```python
from build123d import *

# Parameters (mm, degrees)
ESQUISSE1_R        = 15
ESQUISSE1_R_2      = 3
BOSS_EXTRU_1_DEPTH = 12
CHANFREIN1_SIZE    = 6
CONG_1_R           = 2


with BuildPart() as part:
    # Esquisse1 → Boss.-Extru.1 (new body)
    with BuildSketch(Plane.XY):
        Circle(ESQUISSE1_R)
        Circle(ESQUISSE1_R_2, mode=Mode.SUBTRACT)
    extrude(amount=BOSS_EXTRU_1_DEPTH)

    # Chanfrein1
    chanfrein1_edges = [part.edges().sort_by_distance(p)[0] for p in [
        (-3, 0, 12),
    ]]
    chamfer(chanfrein1_edges, length=CHANFREIN1_SIZE)

    # Congé1
    cong_1_edges = [part.edges().sort_by_distance(p)[0] for p in [
        (-9, 0, 12),
        (-15, 0, 12),
    ]]
    fillet(cong_1_edges, radius=CONG_1_R)


solid = part.part
```
Source: CAD feature listing. Evaluate the final solid. Frame: model axes, mm. Give positions to 0.01 mm unless a question says otherwise; leave off trailing zeros. Order: outer loops, then holes, each group sorted by start corner. A loop starts at its lowest first (then second) coordinate and runs counter-clockwise, first axis right, second up.
(1) Section query D-D (z = 3.25). Return the cut outline in (x, y).
(2) Section query A-A (x = 0). Return the cut outline in (y, z).
(3) Section query C-C (z = 8). Return the cut outline in (x, y).
(4) Material intervals for line 1 along Y through (x, z) = (0, 1.7); line 2 along Z through (x, y) = (-2, 9.5); line 3 along Z through (x, y) = (-4.25, 7.25), sorted ascending.
(5) Contact query for flat-ended pins moving along their axis: P1, Ø4, axis at x = -3, z = 7, coming from the -Y side; P2, Ø3, axis at x = -3, y = -0.5, coming from the +Z side; P3, Ø8, axis at x = 3, y = 2.5, coming from the +Z side. Output: stop coordinate, or through.
(6) Pull-direction query (Y, two-part tool) for faces 1 (the face through (-14.985, 0.66, 4.93)), 2 (the face through (-0.72, -3.26, 6.34)), 3 (the face through (2, 10, 12)); classes: +Y half, -Y half, draft (parallel to the pull), parting line (faces both ways), or undercut.
Outcome:
1. outline: circle Ø30 at (0, 0); hole circle Ø6 at (0, 0)
2. outline: (-15, 0) - (-3, 0) - (-3, 6) - (-8.41, 11.41) arc R2 ccw to (-9.83, 12) - (-13, 12) arc R2 ccw to (-15, 10) - close; (3, 0) - (15, 0) - (15, 10) arc R2 ccw to (13, 12) - (9.83, 12) arc R2 ccw to (8.41, 11.41) - (3, 6) - close
3. outline: circle Ø30 at (0, 0); hole circle Ø10 at (0, 0)
4. line 1: y = -15 to -3, 3 to 15
4. line 2: z = 0 to 12
4. line 3: z = 0 to 11.4
5. P1: stops at y = -14.97
5. P2: stops at z = 7.54
5. P3: stops at z = 10.91
6. face 1: parting line
6. face 2: undercut
6. face 3: draft
